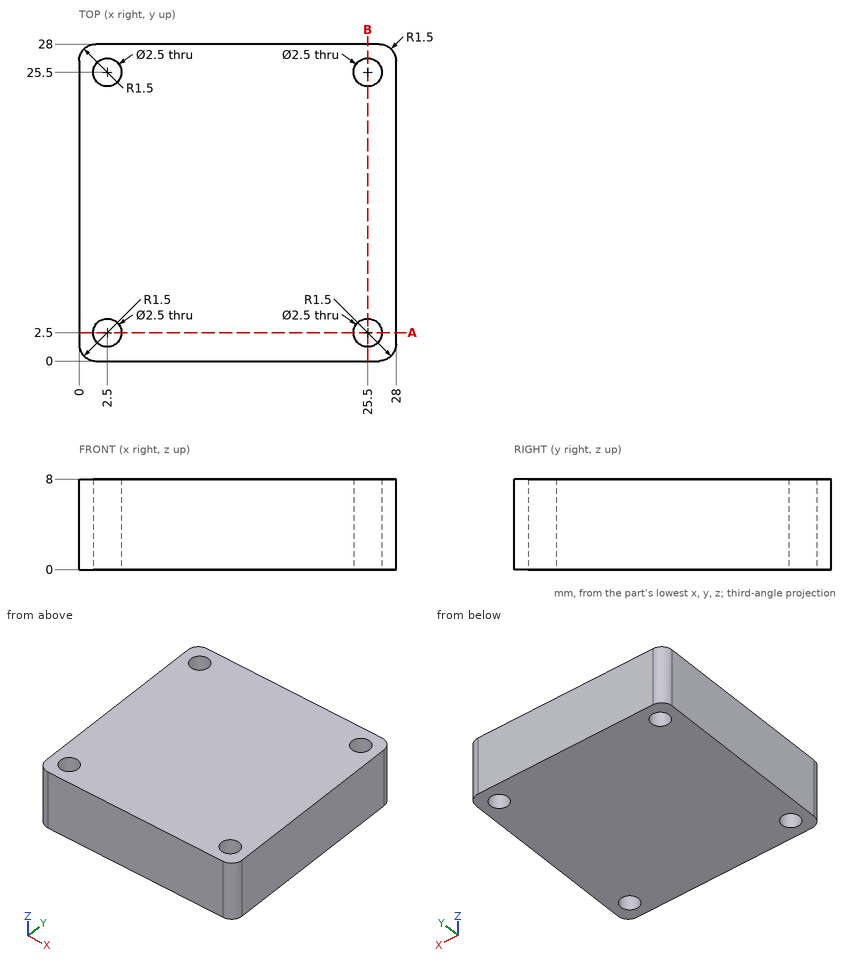
Geometry: see drawing. Coordinates: mm, zero at the bounding-box minimum. Round coordinates to 2 decimals unless told otherwise and drop trailing zeros. Loops run counter-clockwise (first coordinate to the right, second up) from the corner with the lowest first, then second, coordinate; pieces in that order, holes last. Notation, with made-up numbers: M -26,12.25 L -12,12.25 A27 cw -12,49.25 Z; hole C 20.25,81.5 d9. An arc over 180 degrees is marked long. Use a Markdown table: item, result. Add a question column.
1. Ray query, line 1 along Y through (x, z) = (25.5, 5); line 2 along Y through (x, z) = (3.25, 2.75). Return the intervals inside material, ascending. Write a range as [from, to].
2. Cut plane A-A, the plane y = 2.5. Output: boundary loops of the cut face in (x, z).
Solution:
| question | item | result |
|---|---|---|
| 1 | line 1 | y = [0, 1.25], [3.75, 24.25], [26.75, 28] |
| 1 | line 2 | y = [0, 1.5], [3.5, 24.5], [26.5, 28] |
| 2 | outline | M 0,0 L 1.25,0 L 1.25,8 L 0,8 Z; M 3.75,0 L 24.25,0 L 24.25,8 L 3.75,8 Z; M 26.75,0 L 28,0 L 28,8 L 26.75,8 Z |
